Geometry: final body of the model. Coordinates: model frame, mm. A direction names the side the tool comes from. Give positions to 0.01 mm unless a question says otherwise; leave off trailing zeros. Answer as a JSON object with one key per item and string values.
from build123d import *

# Parameters (mm, degrees)
BOSS_EXTRUDE1_DEPTH        = 3
CUT_EXTRUDE1_DEPTH         = 252.974914731
M3_5_CLEARANCE_HOLE1_D     = 3.81
M3_5_CLEARANCE_HOLE1_DEPTH = 33.326039541
FILLET3_R                  = 10
FILLET4_R                  = 4.953107
FILLET10_RADIUS            = 4.717615086
FILLET10_LENGTH            = 3


with BuildPart() as part:
    # Sketch1 → Boss-Extrude1 (new body)
    with BuildSketch(Plane(origin=(-18.747425911, 0, -19.797474517), x_dir=(0, 1, 0), z_dir=(0.6875885279992334, -2.359310851515896e-15, 0.7261005551325845))):
        with BuildLine():
            Line((47.134672347, 186.593127271), (102.029433509, 167.605742926))
            Line((102.029433509, 167.605742926), (110.11778873, 189.999917885))
            add(Edge.make_bspline(
                [(110.11778873, 189.999917885), (95.556778138, 201.958306819), (77.203961524, 210.173231356), (27.942477706, 224.856027605), (-5.55144569, 228.347913352), (-37.305127188, 221.679998311)],
                knots=[0.208168369, 0.208168369, 0.208168369, 0.208168369, 0.5, 0.5, 1, 1, 1, 1], degree=3))
            ThreePointArc((-37.305127188, 221.679998311), (-37.947282057, 219.208911383), (-35.783847857, 217.85311422))
            add(Edge.make_bspline(
                [(48.961630736, 191.875078834), (21.255996477, 223.260445978), (-35.783847857, 217.85311422)],
                knots=[3.106185015, 3.106185015, 3.106185015, 3.3708584, 3.3708584, 3.3708584], degree=2, weights=[1, 0.991256272, 1]))
            Line((48.961630736, 191.875078834), (47.134672347, 186.593127271))
        make_face()
    extrude(amount=-BOSS_EXTRUDE1_DEPTH)

    # Sketch2 → Cut-Extrude1 (cut, through all)
    with BuildSketch(Plane(origin=(-20.810191495, 0, -21.975776182), x_dir=(-0.7261005551325845, -2.234174129215775e-15, 0.6875885279992334), z_dir=(-0.6875885279992334, 2.3593108515158963e-15, -0.7261005551325845))):
        Polygon((170.822075884, 92.730636669), (183.50888872, 56.051568722), (202.112473576, 62.486306908), (189.42566074, 99.165374855), align=None)
    extrude(amount=-CUT_EXTRUDE1_DEPTH, mode=Mode.SUBTRACT)

    # M3.5 Clearance Hole1
    with Locations(Plane(origin=(-18.747425911, 0, -19.797474517), x_dir=(0.7261005551325845, 2.234174129215775e-15, -0.6875885279992334), z_dir=(0.6875885279992334, -2.3593108515158963e-15, 0.7261005551325845))):
        with Locations((-183.058820464, 102.459409082), (-199.141514485, 55.962449256), (-189.875728995, 52.757534495), (-173.793034975, 99.254494321)):
            Hole(M3_5_CLEARANCE_HOLE1_D / 2, depth=M3_5_CLEARANCE_HOLE1_DEPTH)

    # Fillet3
    fillet3_edges = [part.edges().sort_by_distance(p)[0] for p in [
        (-157.737854554, 110.11778873, 109.755138509),
    ]]
    fillet(fillet3_edges, radius=FILLET3_R)

    # Fillet4
    fillet4_edges = [part.edges().sort_by_distance(p)[0] for p in [
        (-141.477431685, 102.029433509, 94.357160713),
        (-143.812812831, 92.730636669, 96.568674357),
    ]]
    fillet(fillet4_edges, radius=FILLET4_R - 0.0001)  # a hair under: the kernel refuses the full size

    # Fillet10: full round fillet: the end face becomes a half cylinder, R = half its width
    fillet10_face = Plane((-154.144448336, 51.593120535, 106.352324843), x_dir=(-0.687588527999, 0, -0.726100555133), z_dir=(0.686211495613, -0.326885353607, -0.649815165171))  # on the end face: x along it, z out of the body
    fillet10_slab = fillet10_face.offset(-FILLET10_RADIUS / 2) * Box(FILLET10_LENGTH, 2 * FILLET10_RADIUS, FILLET10_RADIUS, mode=Mode.PRIVATE)  # the body's end, R deep
    fillet10_round = Plane((-157.38173004, 53.135239811, 109.417902669), x_dir=(0.686211495613, -0.326885353607, -0.649815165171), z_dir=(-0.687588527999, 0, -0.726100555133)) * Cylinder(FILLET10_RADIUS, FILLET10_LENGTH, mode=Mode.PRIVATE)  # its axis R under the face
    add(fillet10_slab - fillet10_round, mode=Mode.SUBTRACT)


solid = part.part
1) Pull-direction query (Z, two-part tool) for faces 4 (the flat face through (-169.47, 45.56, 122.93)), 5 (the cylindrical face through (-179, -38, 130)), 6 (the cylindrical face through (-142.82, 101.21, 95.6)), 7 (the cylindrical face through (-153.4, 100.8, 105.6)); classes: pulls with the +Z half, pulls with the -Z half, needs draft (parallel to the pull), parting line crosses it, or undercut.
Geometry check:
{"face 4": "pulls with the +Z half", "face 5": "parting line crosses it", "face 6": "pulls with the -Z half", "face 7": "undercut"}
2) Contact query for flat-ended pins moving along their axis: P1, Ø8, axis at y = 53, z = 100.5, coming from the -X side; P2, Ø6, axis at x = -167.5, z = 120, coming from the +Y side; P3, Ø2, axis at x = -169.5, y = 46.5, coming from the +Z side. Output: stop coordinate, or through.
Geometry check:
{"P1": "passes through", "P2": "stops at y = 93.76", "P3": "stops at z = 123.91"}
3) Set-up query: faces 1 (the flat face through (-161.34, 60.006, 113.137)), 2 (the flat face through (-171.53, 45.56, 120.75)), 3 (the flat face through (-158.79, 48.82, 110.78)). Return all of +Z, -Z, +X, -X, +Y, -Y with unobstructed straight access to the full face (end or side cutting, diameter ignored); none if empty.
Geometry check:
{"face 1": "-Z, +X", "face 2": "-Z, -X, +Y, -Y", "face 3": "-Y"}
4) Line query: line 1 (Z direction, x = -176.5, y = 57.5); line 2 (Z direction, x = -172.5, y = 59.5); line 3 (Y direction, x = -143.5, z = 97). Output: solid intervals per line, ascending. Write a range as from..to.
Geometry check:
{"line 1": "z = 125.46..127.81", "line 2": "z = 121.67..125.8", "line 3": "y = 95.08..102.98"}
